from build123d import *

# Parameters (mm, degrees)
SKETCH1_W           = 6
SKETCH1_H           = 6
BOSS_EXTRUDE1_DEPTH = 14
HOLE2_D             = 6.4
HOLE2_DEPTH         = 14
HOLE1_D             = 6.4
CUT_EXTRUDE2_DEPTH  = 15
CUT_EXTRUDE1_DEPTH  = 27.088457268
SKETCH8_R           = 3.15
CUT_EXTRUDE3_DEPTH  = 15


with BuildPart() as part:
    # Sketch1 → Boss-Extrude1 (new body)
    with BuildSketch(Plane.XY.offset(14)):
        with BuildLine():
            Line((7, 0), (7, 20.267949192))
            Line((7, 20.267949192), (2, 28.92820323))
            Line((2, 28.92820323), (-15.552558883, 39.062177826))
            ThreePointArc((-15.552558883, 39.062177826), (-25.11473671, 36.5), (-22.552558883, 26.937822174))
            Line((-22.552558883, 26.937822174), (-10.464101615, 19.958548116))
            Line((-10.464101615, 19.958548116), (-7, 13.958548116))
            Line((-7, 13.958548116), (-7, 0))
            ThreePointArc((-7, 0), (-6.480740698, -2.645751311), (-5, -4.898979486))
            Line((-5, -4.898979486), (-5, -14))
            Line((-5, -14), (-6, -14))
            Line((-6, -14), (-6, -16))
            Line((-6, -16), (6, -16))
            Line((6, -16), (6, -14))
            Line((6, -14), (5, -14))
            Line((5, -14), (5, -4.898979486))
            ThreePointArc((5, -4.898979486), (6.480740698, -2.645751311), (7, 0))
        make_face()
        with Locations((0, -11)):
            Rectangle(SKETCH1_W, SKETCH1_H, mode=Mode.SUBTRACT)
    extrude(amount=-BOSS_EXTRUDE1_DEPTH)

    # Hole2
    with Locations(Plane(origin=(0, 0, 0), x_dir=(-1, 0, 0), z_dir=(0, 0, -1))):
        with Locations((19.0525, 32.999898011)):
            Hole(HOLE2_D / 2, depth=HOLE2_DEPTH)

    # Hole1 (through all)
    with Locations(Plane(origin=(0, 0, 0), x_dir=(-1, 0, 0), z_dir=(0, 0, -1))):
        with Locations((0, 0)):
            Hole(HOLE1_D / 2)

    # Sketch3 → Cut-Extrude2 (cut, through all)
    with BuildSketch(Plane.ZY.offset(7)):
        with BuildLine():
            Line((9.2627417, 4.7372583), (11.5254834, 7))
            Line((11.5254834, 7), (9.2627417, 9.2627417))
            ThreePointArc((9.2627417, 9.2627417), (3.8, 7), (9.2627417, 4.7372583))
        make_face()
    extrude(amount=-CUT_EXTRUDE2_DEPTH, mode=Mode.SUBTRACT)

    # Sketch2 → Cut-Extrude1 (cut, through all)
    with BuildSketch(Plane(origin=(6.026279442, 10.437822174, 0), x_dir=(0.866025404, -0.5, 0), z_dir=(-0.5, -0.866025404, 0))):
        with BuildLine():
            Line((-25.999898011, 11.5254834), (-28.262639711, 9.2627417))
            ThreePointArc((-28.262639711, 9.2627417), (-25.999898011, 3.8), (-23.737156311, 9.2627417))
            Line((-23.737156311, 9.2627417), (-25.999898011, 11.5254834))
        make_face()
    extrude(amount=-CUT_EXTRUDE1_DEPTH, mode=Mode.SUBTRACT)

    # Sketch8 → Cut-Extrude3 (cut, through all)
    with BuildSketch(Plane.XY.offset(14)):
        with Locations((-2.116025404, 20.778312164)):
            Circle(SKETCH8_R)
    extrude(amount=-CUT_EXTRUDE3_DEPTH, mode=Mode.SUBTRACT)


solid = part.part
Geometry: final body of the model. Coordinates: model frame, mm. A direction names the side the tool comes from. Give positions to 0.01 mm unless a question says otherwise; leave off trailing zeros. Loops run counter-clockwise (first coordinate to the right, second up) from the corner with the lowest first, then second, coordinate; pieces in that order, holes last. Notation, with made-up numbers: M 57,9.5 L 79,9.5 A18 cw 79,22.5 Z; hole C 29,8 d11. An arc over 180 degrees is marked long. Put each result on its own line as item: value. Start each with the question number.
1) Cut plane B-B (x = 0). Output: boundary loops of the cut face in (y, z).
2) Cut plane C-C (x = 4). Output: boundary loops of the cut face in (y, z).
3) Ray query, line 1 along Y through (x, z) = (0, 10.75); line 2 along Y through (x, z) = (2, 9.25); line 3 along Y through (x, z) = (0, 10.25). Return the intervals inside material, ascending.
4) Access query for faces 4 (the flat face through (3, -11, 7)), 5 (the cylindrical face through (-6.5, -2.6, 7.1)), 6 (the flat face through (-0.098, 5.853, 10.378)), 7 (the cylindrical face through (6.466, -2.681, 7.098)). Directions: +Z, -Z, +X, -X, +Y, -Y. A direction counts if a zero-diameter tool reaches every point of the face in a straight line with its end or side. Return the directions, or none.
5) Cut plane A-A (z = 4.5). Give the number of separate pieces and of enclosed holes in the cut face, then the cut area to 3 significant figures.
6) Contact query for flat-ended pins moving along their axis: pin 1 (4 mm diameter, centred on y = 7, z = 7, fed in from +X); pin 2 (2 mm diameter, centred on y = -15.5, z = 9.5, fed in from -X); pin 3 (3 mm diameter, centred on y = -10.5, z = 8.5, fed in from +X); pin 4 (1.8 mm diameter, centred on y = -10.5, z = 5.5, fed in from -X). Output: stop coordinate, or through.
7) Cut plane D-D (y = 1). Output: boundary loops of the cut face in (x, z).
8) Pull-direction query (Z, two-part tool) for faces 1 (the flat face through (-6, 19, 14)), 2 (the flat face through (-12.05, 28.84, 10.38)), 3 (the flat face through (-8.756, 17.001, 7.098)); classes: pulls with the +Z half, pulls with the -Z half, needs draft (parallel to the pull), parting line crosses it, or undercut.
Verdict:
1. outline: M -16,0 L -14,0 L -14,14 L -16,14 Z; M -8,0 L -3.2,0 L -3.2,14 L -8,14 Z; M 3.2,0 L 18.44,0 L 18.44,14 L 3.2,14 Z; M 23.11,0 L 30.08,0 L 30.08,14 L 23.11,14 Z; hole M 4.74,9.26 A3.2 ccw long 9.26,9.26 L 7,11.53 Z
2. outline: M -16,0 L 25.46,0 L 25.46,14 L -16,14 Z; hole M 4.74,9.26 A3.2 ccw long 9.26,9.26 L 7,11.53 Z
3. line 1: -16 to -14, -8 to -3.2, 3.2 to 6.22, 7.78 to 18.44, 23.11 to 30.08
3. line 2: -16 to -14, -8 to -2.5, 2.5 to 4.72, 9.28 to 28.93
3. line 3: -16 to -14, -8 to -3.2, 3.2 to 5.72, 8.28 to 18.44, 23.11 to 30.08
4. face 4: +Z, -Z
4. face 5: +Z, -Z, -X
4. face 6: +X, -X
4. face 7: +Z, -Z, +X
5. separate pieces: 3
5. enclosed holes: 4
5. area: 620 mm2
6. pin 1: through
6. pin 2: x = -6
6. pin 3: x = 5
6. pin 4: x = -5
7. outline: M -7,0 L -3.04,0 L -3.04,14 L -7,14 Z; M 3.04,0 L 7,0 L 7,14 L 3.04,14 Z
8. face 1: pulls with the +Z half
8. face 2: undercut
8. face 3: needs draft
